from build123d import *

# Parameters (mm, degrees)
SKETCH1_W           = 46.896511464
SKETCH1_H           = 46.896511464
SKETCH1_W_2         = 43.412298388
SKETCH1_H_2         = 43.412298388
BOSS_EXTRUDE1_DEPTH = 1.5
SKETCH1_3_W         = 49.664280744
SKETCH1_3_H         = 49.664280744
SKETCH1_3_W_2       = 46.896511464
SKETCH1_3_H_2       = 46.896511464
BOSS_EXTRUDE2_DEPTH = 3.5
BOSS_EXTRUDE4_START = -3.5
SKETCH2_R           = 3.75
SKETCH2_R_2         = 1.5
BOSS_EXTRUDE4_DEPTH = 8.5
FILLET2_R           = 3


with BuildPart() as part:
    # Sketch1 → Boss-Extrude1 (new body)
    with BuildSketch(Plane(origin=(0, 0, 0), x_dir=(1, 0, 0), z_dir=(0, 1, 0))):
        Rectangle(SKETCH1_W, SKETCH1_H)
        Rectangle(SKETCH1_W_2, SKETCH1_H_2, mode=Mode.SUBTRACT)
    extrude(amount=BOSS_EXTRUDE1_DEPTH)

    # Sketch1<3> → Boss-Extrude2 (add)
    with BuildSketch(Plane(origin=(0, 0, 0), x_dir=(1, 0, 0), z_dir=(0, 1, 0))):
        Rectangle(SKETCH1_3_W, SKETCH1_3_H)
        Rectangle(SKETCH1_3_W_2, SKETCH1_3_H_2, mode=Mode.SUBTRACT)
    extrude(amount=BOSS_EXTRUDE2_DEPTH)

    # Sketch2 → Boss-Extrude4 (add)
    # profile 1 of 2: a face of its own
    with BuildSketch(Plane(origin=(0, 3.5, 0), x_dir=(1, 0, 0), z_dir=(0, 1, 0)).offset(BOSS_EXTRUDE4_START)):
        with Locations(Location((-28.332140372, 9.832140372, 0), (0, 0, 270))):
            Circle(SKETCH2_R)
        with Locations(Location((-28.332140372, 9.832140372, 0), (0, 0, 270))):
            Circle(SKETCH2_R_2, mode=Mode.SUBTRACT)
    # profile 2 of 2: a face of its own
    with BuildSketch(Plane(origin=(0, 3.5, 0), x_dir=(1, 0, 0), z_dir=(0, 1, 0)).offset(BOSS_EXTRUDE4_START)):
        with Locations(Location((28.332140372, 9.832140372, 0), (0, 0, 201.039469781))):
            Circle(SKETCH2_R)
        with Locations(Location((28.332140372, 9.832140372, 0), (0, 0, 270))):
            Circle(SKETCH2_R_2, mode=Mode.SUBTRACT)
    extrude(amount=BOSS_EXTRUDE4_DEPTH)

    # Fillet2
    fillet2_edges = [part.edges().sort_by_distance(p)[0] for p in [
        (-24.832140372, 1.75, -8.48584917),
        (-24.832140372, 1.75, -11.178431574),
        (24.832140372, 1.75, -8.48584917),
        (24.832140372, 1.75, -11.178431574),
    ]]
    fillet(fillet2_edges, radius=FILLET2_R)


solid = part.part
Input: part model. Units: mm. Frame: model coordinates. A direction names the side the tool comes from. Coordinates: 2 decimals unless noted, no trailing zeros. Loops run counter-clockwise (first coordinate to the right, second up) from the corner with the lowest first, then second, coordinate; pieces in that order, holes last. Notation, with made-up numbers: (25.5, -7) -> (76.5, -7) arc R3 ccw to (76.5, -2) -> close; hole circle Ø9 at (14.5, -34). An arc over 180 degrees is marked (long way). Write each question's results on one line, items separated by ' | '. Start each with the question number.
Q1. Section C-C, the plane y = 2.5. Return the cut outline in (x, z).
Q2. Section A-A, the plane z = 3. Return the cut outline in (x, y).
Q3. Section B-B, the plane x = 18. Return the cut outline in (y, z), plus the area to 3 significant figures.
Q4. Ray query, line 1 (X direction, y = 2, z = -19); line 2 (X direction, y = 1, z = 5.5). Return the intervals inside material, ascending. Write a range as from..to.
Q5. Pin query (flat end, axial travel): pin 1 (5 mm diameter, centred on y = 5.5, z = -0.5, fed in from +X); pin 2 (12 mm diameter, centred on x = 6, z = -18.5, fed in from +Y); pin 3 (2 mm diameter, centred on y = 2, z = -11.5, fed in from +X); pin 4 (5 mm diameter, centred on x = 28.33, z = -9.83, fed in from -Y). Return the tip coordinate at first contact, or that it passes through.
Q6. Pull-direction query (Z, two-part tool) for faces 1 (the flat face through (23.448, 2, 0)), 2 (the cylindrical face through (25.816, 1.774, -5.323)), 3 (the flat face through (0, 0, -22)); classes: released by +Z, released by -Z, zero draft, split by the parting line, or undercut.
Q7. Reachability of faces 4 (the flat face through (-2, 1.5, 22)), 5 (the flat face through (24.832, 2, 11)), 6 (the flat face through (24.832, 2, -21)), 7 (the flat face through (-24.832, 2, 11)), 8 (the flat face through (-21.706, 1, 0)) from +Z, -Z, +X, -X, +Y, -Y: full face, straight path, thin tool, end or side. Return the list, or none.
Found:
1) outline: (-28.05, -13.57) arc R3 cw to (-24.83, -16.56) -> (-24.83, -24.83) -> (24.83, -24.83) -> (24.83, -16.56) arc R3 cw to (28.05, -13.57) arc R3.75 ccw (long way) to (28.05, -6.09) arc R3 cw to (24.83, -3.1) -> (24.83, 24.83) -> (-24.83, 24.83) -> (-24.83, -3.1) arc R3 cw to (-28.05, -6.09) arc R3.75 ccw (long way) to start; hole circle Ø3 at (-28.33, -9.83); hole (-23.45, -23.45) -> (23.45, -23.45) -> (23.45, 23.45) -> (-23.45, 23.45) -> close; hole circle Ø3 at (28.33, -9.83)
2) outline: (-24.83, 0) -> (-21.71, 0) -> (-21.71, 1.5) -> (-23.45, 1.5) -> (-23.45, 3.5) -> (-24.83, 3.5) -> close; (21.71, 0) -> (24.83, 0) -> (24.83, 3.5) -> (23.45, 3.5) -> (23.45, 1.5) -> (21.71, 1.5) -> close
3) outline: (0, -24.83) -> (3.5, -24.83) -> (3.5, -23.45) -> (1.5, -23.45) -> (1.5, -21.71) -> (0, -21.71) -> close; (0, 21.71) -> (1.5, 21.71) -> (1.5, 23.45) -> (3.5, 23.45) -> (3.5, 24.83) -> (0, 24.83) -> close | area: 14.9 mm2
4) line 1: -24.83..-23.45, 23.45..24.83 | line 2: -24.83..-21.71, 21.71..24.83
5) pin 1: x = 24.83 | pin 2: y = 3.5 | pin 3: x = 32.02 | pin 4: y = 0
6) face 1: undercut | face 2: released by +Z | face 3: zero draft
7) face 4: +Y | face 5: +Z, +X, +Y, -Y | face 6: -Z, +X, +Y, -Y | face 7: +Z, -X, +Y, -Y | face 8: +Y, -Y
